CAD build for the part. Positions are in the model's coordinates, mm. Round coordinates to 2 decimals unless told otherwise and drop trailing zeros. Loops run counter-clockwise (first coordinate to the right, second up) from the corner with the lowest first, then second, coordinate; pieces in that order, holes last.
```python
from build123d import *

# Parameters (mm, degrees)
F0_R     = 7.5
F0_R_2   = 4.5
F1_DEPTH = 42.5
F2_R     = 1.5


with BuildPart() as f1:
    # F0 (on Right) → F1 (new body)
    with BuildSketch(Plane.YZ):
        Circle(F0_R)
        Circle(F0_R_2, mode=Mode.SUBTRACT)
    extrude(amount=F1_DEPTH)

    # F2
    f2_edges = [f1.edges().sort_by_distance(p)[0] for p in [
        (42.5, -7.5, 0),
        (0, -7.5, 0),
    ]]
    fillet(f2_edges, radius=F2_R)

    # F6 (on Front) → F7 (revolve, cut)
    with BuildSketch(Plane.XZ):
        Polygon((5.414214, 8.414214), (2.585786, 8.414214), (4, 7), align=None)
        Polygon((6.410786, 8.414214), (7.825, 7), (9.239214, 8.414214), align=None)
        Polygon((10.235786, 8.414214), (11.65, 7), (13.064214, 8.414214), align=None)
        Polygon((14.060786, 8.414214), (15.475, 7), (16.889214, 8.414214), align=None)
        Polygon((17.885786, 8.414214), (19.3, 7), (20.714214, 8.414214), align=None)
        Polygon((21.710786, 8.414214), (23.125, 7), (24.539214, 8.414214), align=None)
        Polygon((25.535786, 8.414214), (26.95, 7), (28.364214, 8.414214), align=None)
        Polygon((29.360786, 8.414214), (30.775, 7), (32.189214, 8.414214), align=None)
        Polygon((33.185786, 8.414214), (34.6, 7), (36.014214, 8.414214), align=None)
        Polygon((37.010786, 8.414214), (38.425, 7), (39.839214, 8.414214), align=None)
    revolve(axis=Axis((21.25, 0, 0), (1, 0, 0)), mode=Mode.SUBTRACT)


solid = f1.part
```
Item 1: Probe line 1 (Z direction, x = 26, y = 0); line 2 (Y direction, x = 14.5, z = 1); line 3 (X direction, y = 3.75, z = -4.75). List the from-to ranges inside material, lowest first.
Answers follow:
line 1: z = -7.5 to -4.5, 4.5 to 7.5
line 2: y = -7.43 to -4.39, 4.39 to 7.43
line 3: x = 0 to 42.5
Item 2: Cut at A-A, the plane x = 3. Give the cut face in (y, z), plus the area to 3 significant figures.
Answers follow:
outline: circle Ø15 at (0, 0); hole circle Ø9 at (0, 0)
area: 113 mm2
Item 3: Flat gauge pins, fed straight in: P1, Ø2, axis at x = 19, y = 1.5, coming from the +Z side; P2, Ø3, axis at x = 28.5, y = -2, coming from the -Z side; P3, Ø2, axis at y = -3, z = 0.5, coming from the -X side; P4, Ø5, axis at x = 6, y = 3.5, coming from the -Z side. Where does each tip first touch, or does it go through?
Answers follow:
P1: stops at z = 7.48
P2: stops at z = -7.48
P3: passes through
P4: stops at z = -7.43
